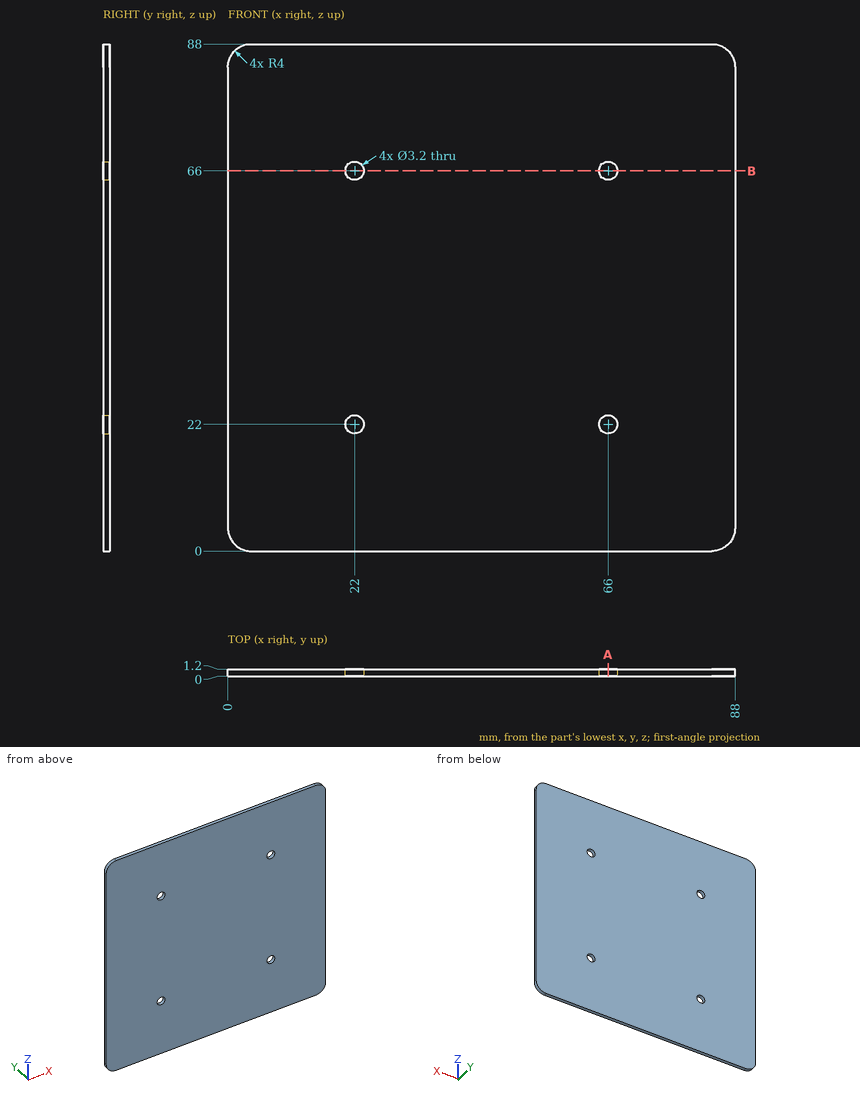
Verification items for this drawing (mm, ordinates from the low corner). Coordinates: 2 decimals unless noted, no trailing zeros. Order: outer loops, then holes, each group sorted by start corner. A loop starts at its lowest first (then second) coordinate and runs counter-clockwise, first axis right, second up. Notation, with made-up numbers: M 70.5,74 L 100.5,74 A18 cw 100.5,82 Z; hole C 11,-6 d9. An arc over 180 degrees is marked long. One line per item, written item: value. Start each with the question number.
Item 1: Sectioned sample at B-B on z = 66. Record the cut outline in (x, y), then the cut area to 3 significant figures.
Item 2: Thickness scan on probe 1 along X at (y, z) = (0.5, 66). Record the ranges inside material, lowest first.
Item 3: Sectioned sample at A-A on x = 66. Record the cut outline in (y, z).
Item 4: Depth check by flat-ended pin: P1, Ø2.5, axis at x = 66, z = 22, coming from the +Y side. Enter the tip coordinate at first touch or a pass-through.
Calculated:
1. outline: M 0,0 L 20.4,0 L 20.4,1.2 L 0,1.2 Z; M 23.6,0 L 64.4,0 L 64.4,1.2 L 23.6,1.2 Z; M 67.6,0 L 88,0 L 88,1.2 L 67.6,1.2 Z
1. area: 97.9 mm^2
2. probe 1: 0 to 20.4, 23.6 to 64.4, 67.6 to 88
3. outline: M 0,0 L 1.2,0 L 1.2,20.4 L 0,20.4 Z; M 0,23.6 L 1.2,23.6 L 1.2,64.4 L 0,64.4 Z; M 0,67.6 L 1.2,67.6 L 1.2,88 L 0,88 Z
4. P1: through
